Check sheet for the drawn part. Datum: minimum x, y, z corner. Units: mm. Give positions to 0.01 mm unless a question says otherwise; leave off trailing zeros. Order: outer loops, then holes, each group sorted by start corner. A loop starts at its lowest first (then second) coordinate and runs counter-clockwise, first axis right, second up. Notation, with made-up numbers: (35.5, -18) -> (84.5, -18) arc R27 ccw to (84.5, 15) -> close; hole circle Ø1 at (8.25, -18.5). An arc over 180 degrees is marked (long way). One line per question, with ' | ' between items. Start each with the question number.
Q1. Go/stop test with a flat-tipped pin: pin 1 (1.5 mm diameter, centred on y = 3, z = 2.5, fed in from -X). Record where the tip stops, or that it passes through.
Q2. Section check A-A on z = 1.1. Record the cut outline in (x, y), plus the area to 3 significant figures.
Q3. Material ranges on probe 1 along X at (y, z) = (3, 2.3); probe 2 along X at (y, z) = (5.5, 2.75); probe 3 along Y at (x, z) = (4, 2.75), recorded low to high. Write a range as [from, to].
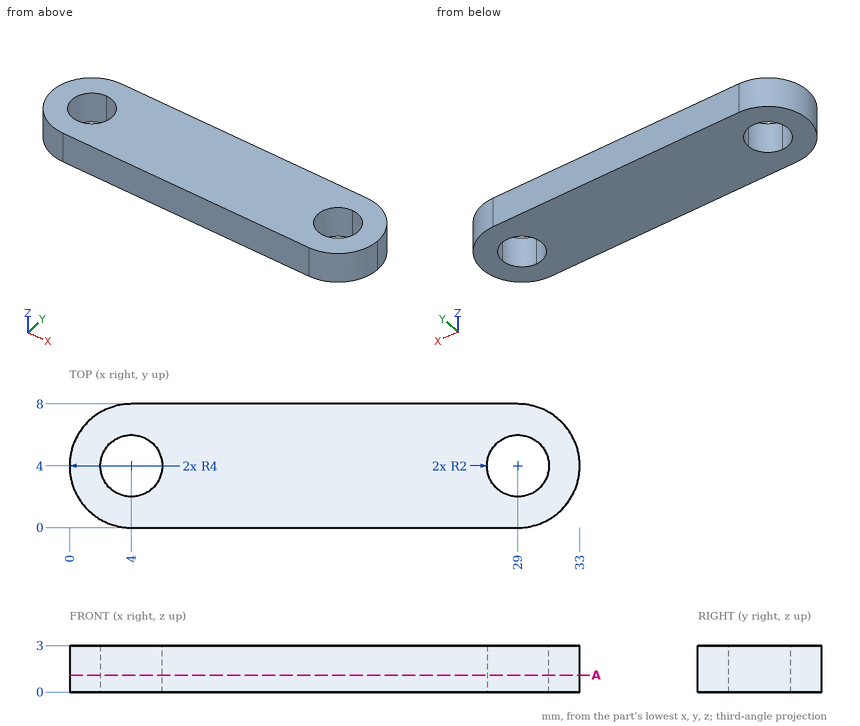
Filled in:
1) pin 1: x = 0.01
2) outline: (4, 0) -> (29, 0) arc R4 ccw to (29, 8) -> (4, 8) arc R4 ccw to start; hole circle Ø4 at (4, 4); hole circle Ø4 at (29, 4) | area: 225 mm²
3) probe 1: [0.13, 2.27], [5.73, 27.27], [30.73, 32.87] | probe 2: [0.29, 2.68], [5.32, 27.68], [30.32, 32.71] | probe 3: [0, 2], [6, 8]
